Design review of the part built by this model. Coordinates are the model's own, in mm. Give positions to 0.01 mm unless a question says otherwise; leave off trailing zeros. Loops run counter-clockwise (first coordinate to the right, second up) from the corner with the lowest first, then second, coordinate; pieces in that order, holes last. Notation, with made-up numbers: (7, -23.5) - (17, -23.5) arc R23 ccw to (17, -12.5) - close; hole circle Ø2 at (30.25, -21.75). An arc over 180 degrees is marked (long way). One line per item, written item: value. Start each with the question number.
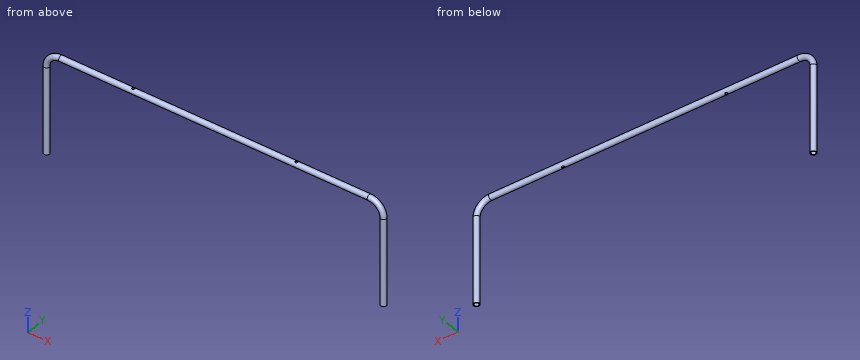
```python
from build123d import *

# Parameters (mm, degrees)
F1_R     = 12.7
F1_R_2   = 9.525
F4_R     = 6.35
F5_DEPTH = 12.7


with BuildPart() as f2:
    # F2: sweep along a path in F0
    with BuildLine(Plane.XZ) as f2_path:
        Line((-752.475, 0), (-752.475, 393.7))
        ThreePointArc((-752.475, 393.7), (-733.8762806053, 438.6012806053), (-688.975, 457.2))
        Line((-688.975, 457.2), (688.975, 457.2))
        ThreePointArc((688.975, 457.2), (733.8762806053, 438.6012806053), (752.475, 393.7))
        Line((752.475, 393.7), (752.475, 0))
    # F1 (on Top) → F2 (sweep)
    with BuildSketch(Plane.XY):
        with Locations((-752.475, 0)):
            Circle(F1_R)
        with Locations((-752.475, 0)):
            Circle(F1_R_2, mode=Mode.SUBTRACT)
    sweep(path=f2_path.line)

    # F4 (on offset) → F5 (cut, symmetric)
    with BuildSketch(Plane.XY.offset(457.2)):
        with Locations((-364.49, 0)):
            Circle(F4_R)
        with Locations((364.49, 0)):
            Circle(F4_R)
    extrude(amount=F5_DEPTH, both=True, mode=Mode.SUBTRACT)


solid = f2.part
```
(1) Take a section at C-C on y = 0. State how many separate pieces and enclosed holes the cut face has, and give its area (3 significant figures).
(2) Take a section at A-A on z = 279.5. State the section outline as (x, y) points (3 decimals).
(3) To check wall thickness, follow L1, parallel to X at y = -2, z = 85.5; L2, parallel to Z at x = -277.5, y = 1; L3, parallel to X at y = -8, z = 115.5. State the ranges of each line that lie inside material, in increasing order. Write a range as from..to.
(4) Take a section at B-B on x = -71.5. State the section outline as (y, z) points (3 decimals), and give its area (3 significant figures).
(5) For pin 1 Ø2 at (x, y) = (-230.5, -10) entering from -Z; pin 2 Ø3 at (y, z) = (8, 317) entering from +X; pin 3 Ø1.5 at (x, y) = (-248, -9) entering from -Z; pin 4 Ø11.5 at (x, y) = (364.49, 0) entering from +Z, all flat-tipped, find the tip position at first contact; note any pin that passes through.
Here are the results:
1. separate pieces: 6
1. enclosed holes: 0
1. area: 14,900 mm²
2. outline: circle Ø25.4 at (-752.475, 0); circle Ø25.4 at (752.475, 0); hole circle Ø19.05 at (-752.475, 0); hole circle Ø19.05 at (752.475, 0)
3. L1: -765.02..-761.79, -743.16..-739.93, 739.93..743.16, 761.79..765.02
3. L2: 444.54..447.73, 466.67..469.86
3. L3: -762.34..-757.64, -747.31..-742.61, 742.61..747.31, 757.64..762.34
4. outline: circle Ø25.4 at (0, 457.2); hole circle Ø19.05 at (0, 457.2)
4. area: 222 mm²
5. pin 1: z = 448.24
5. pin 2: x = 763.39
5. pin 3: z = 447.54
5. pin 4: through
